from build123d import *

# Parameters (mm, degrees)
F1_DEPTH = 7
F2_R     = 3
F3_W     = 0.695917
F3_H     = 7
F4_DEPTH = 2


with BuildPart() as f1:
    # F0 (on Front) → F1 (new body)
    with BuildSketch(Plane.XZ):
        Polygon((0, 9), (0, 6), (2, 6), (4, 9), align=None)
        Polygon((2, 6), (0, 6), (0, 0), (4, 0), (4, 2), (2, 2), (2, 4), (56, 4), (56, 2), (54, 2), (54, 0), (58, 0), (58, 6), (56, 6), align=None)
        Polygon((54, 9), (56, 6), (58, 6), (58, 9), align=None)
    extrude(amount=F1_DEPTH)

    # F2
    f2_edges = [f1.edges().sort_by_distance(p)[0] for p in [
        (0, -3.5, 9),
        (58, -3.5, 9),
    ]]
    fillet(f2_edges, radius=F2_R)

    # F3 (on face) → F4 (join)
    with BuildSketch(Plane(origin=(0, 0, 4), x_dir=(1, 0, 0), z_dir=(0, 0, -1))):
        with Locations((29.347958, 3.5)):
            Rectangle(F3_W, F3_H)
    extrude(amount=F4_DEPTH)


solid = f1.part
Read the model definition and answer for the solid it produces. Units are mm, in the model's axes. A direction names the side the tool comes from. Give positions to 0.01 mm unless a question says otherwise; leave off trailing zeros. Write each loop counter-clockwise with the first axis right and the second up, starting at its lowest first coordinate (ties: lowest second). Pieces come first, ordered by that corner, then holes. Notation, with made-up numbers: M 28,6 L 76,6 A21 cw 76,22 Z; hole C 78,39 d9. An arc over 180 degrees is marked long. One line per item, written item: value. Start each with the question number.
(1) Flat-ended cylindrical pins translate along their axes: pin 1 Ø3.5 at (x, y) = (46.5, -5) entering from -Z; pin 2 Ø2 at (y, z) = (-6, 8) entering from -X; pin 3 Ø0.6 at (x, y) = (29.5, -2.5) entering from -Z. Find the tip coordinate at first contact, or state that the pin passes through.
(2) Find section B-B (y = -2). Determine the outline of the cut face in (x, z).
(3) Find section C-C (z = 8.25). Determine the outline of the cut face in (x, y), plus the area to 3 significant figures.
(4) Find section A-A (z = 0.5). Determine the outline of the cut face in (x, y).
(5) Find section D-D (x = 26.5). Determine the outline of the cut face in (y, z).
(6) Determine the mould class of faces 1 (the flat face through (58, -3, 3)), 2 (the flat face through (54, -3, 1)), 3 (the flat face through (29, -7, 5)) for opening direction X: pulls with the +X half, pulls with the -X half, needs draft (parallel to the pull), parting line crosses it, or undercut.
(7) A tool of negligible diameter and unlimited length cuts with its end or side. For faces 4 (the flat face through (29.696, -3, 3)), 5 (the flat face through (2, -3, 3)), 6 (the flat face through (54.5, -3.5, 9)), from which of +Z, -Z, +X, -X, +Y, -Y can it reach the whole face along a straight path? Write none if from no direction.
(8) Find the intervals of material crossed by line 1 (X direction, y = -0.5, z = 2.5); line 2 (X direction, y = -4, z = 1.5); line 3 (Z direction, x = 17.5, y = -1.75), in increasing order.
Results below:
1. pin 1: stops at z = 4
1. pin 2: stops at x = 0.17
1. pin 3: stops at z = 2
2. outline: M 0,0 L 4,0 L 4,2 L 2,2 L 2,4 L 29,4 L 29,2 L 29.7,2 L 29.7,4 L 56,4 L 56,2 L 54,2 L 54,0 L 58,0 L 58,6 A3 ccw 55,9 L 54,9 L 56,6 L 2,6 L 4,9 L 3,9 A3 ccw 0,6 Z
3. outline: M 1.02,-7 L 3.5,-7 L 3.5,0 L 1.02,0 Z; M 54.5,-7 L 56.98,-7 L 56.98,0 L 54.5,0 Z
3. area: 34.8 mm^2
4. outline: M 0,-7 L 4,-7 L 4,0 L 0,0 Z; M 54,-7 L 58,-7 L 58,0 L 54,0 Z
5. outline: M -7,4 L 0,4 L 0,6 L -7,6 Z
6. face 1: pulls with the +X half
6. face 2: undercut
6. face 3: needs draft
7. face 4: -Z, +Y, -Y
7. face 5: +Y, -Y
7. face 6: +Z, +X, -X, +Y, -Y
8. line 1: x = 0 to 2, 29 to 29.7, 56 to 58
8. line 2: x = 0 to 4, 54 to 58
8. line 3: z = 4 to 6
